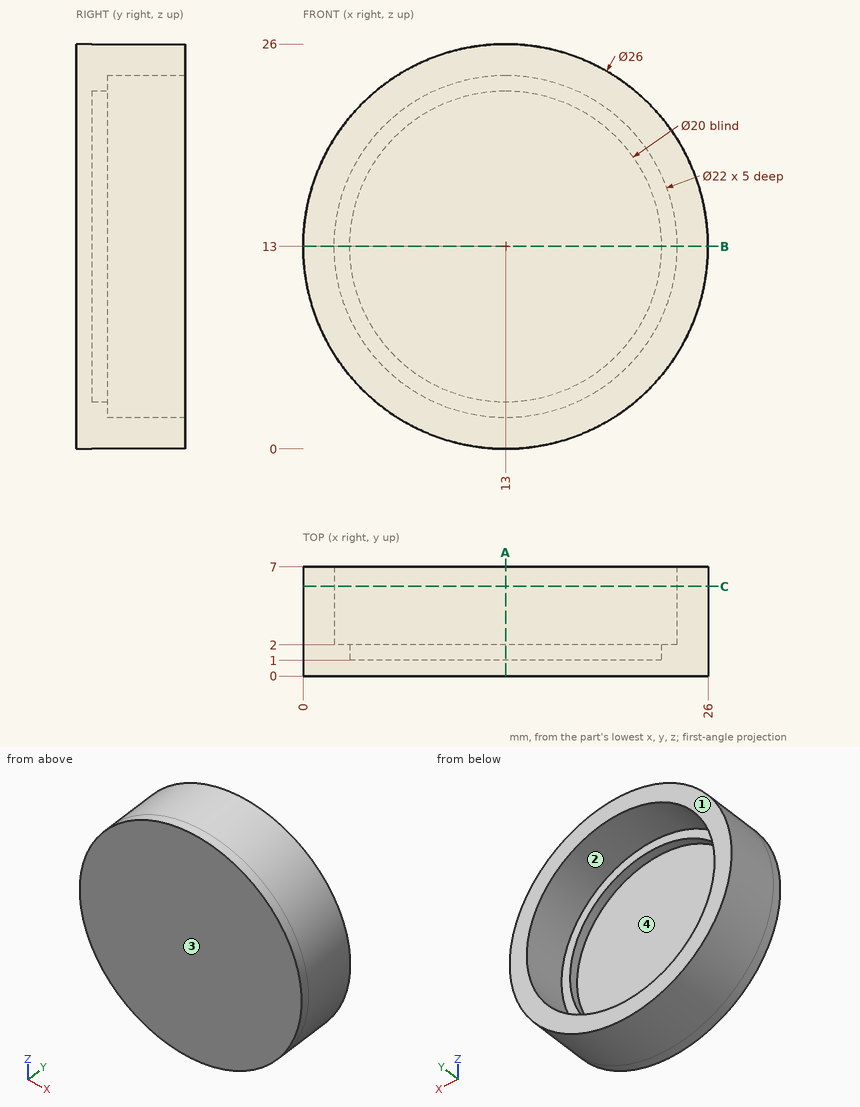
Design review of the part shown in the three views and the two pictorial views. Dimensions are in mm from the part's minimum x, y and z. A direction names the side the tool comes from. Round coordinates to 2 decimals unless told otherwise and drop trailing zeros. Write each loop counter-clockwise with the first axis right and the second up, starting at its lowest first coordinate (ties: lowest second). Pieces come first, ordered by that corner, then holes. Notation, with made-up numbers: (74, 56.5) -> (129, 56.5) arc R14 ccw to (129, 72.5) -> close; hole circle Ø11 at (22, -25.75). An arc over 180 degrees is marked (long way). One line per question, with ' | ' between items. Start each with the question number.
1) Add section B-B (z = 13). Write out the cut boundary in (x, y), and give its area (3 significant figures).
2) For pin 1 Ø2 at (y, z) = (5.5, 4.5) entering from -X; pin 2 Ø12 at (x, z) = (13.5, 11.5) entering from +Y; pin 3 Ø1 at (y, z) = (5, 15) entering from +X, all flat-tipped, find the tip position at first contact; note any pin that passes through.
3) Machinability: for the marked faces 3 and 4, which of the approach directions +Z, -Z, +X, -X, +Y, -Y give a long, thin tool a straight path to every point of the face, cutting with its end or side? Answer none if there is none.
4) Mouldability with a two-part tool opening along X and no side actions: class the marked faces 1 and 2 as +X half, -X half, draft (parallel to the pull), parting line (faces both ways), or undercut.
5) Wall thickness on line 1 along X through (y, z) = (5, 12.75); line 2 along X through (y, z) = (1.5, 13); line 3 along Y through (x, z) = (2.75, 16): over which ranges is each line inside the solid? List them lowest first.
6) Add section A-A (x = 13). Write out the cut boundary in (y, z), and give its area (3 significant figures).
7) Add section C-C (y = 5.75). Write out the cut boundary in (x, z), and give its area (3 significant figures).
Reported:
1) outline: (0, 0) -> (26, 0) -> (26, 7) -> (24, 7) -> (24, 2) -> (23, 2) -> (23, 1) -> (3, 1) -> (3, 2) -> (2, 2) -> (2, 7) -> (0, 7) -> close | area: 52.0 mm²
2) pin 1: stops at x = 2.38 | pin 2: stops at y = 1 | pin 3: stops at x = 25.91
3) face 3: +Z, -Z, +X, -X, -Y | face 4: +Y
4) face 1: draft | face 2: undercut
5) line 1: x = 0 to 2, 24 to 26 | line 2: x = 0 to 3, 23 to 26 | line 3: y = 0 to 2
6) outline: (0, 0) -> (7, 0) -> (7, 2) -> (2, 2) -> (2, 3) -> (1, 3) -> (1, 23) -> (2, 23) -> (2, 24) -> (7, 24) -> (7, 26) -> (0, 26) -> close | area: 52.0 mm²
7) outline: circle Ø26 at (13, 13); hole circle Ø22 at (13, 13) | area: 151 mm²
